Solid Edge part; units mm, degrees
sketch "Sketch1" plane through (0, 0, 0) normal (0, -1, 0) x (1, 0, 0)
  line L0 (-7, -6) -> (7, -6)
  line L1 (7, -6) -> (7, 6)
  line L2 (7, 6) -> (-7, 6)
  line L3 (-7, 6) -> (-7, -6)
  dimension "D1" = 7
  dimension "D2" = 7
extrude "Protrusion1" add sketch "Sketch1" along normal blind 40
sketch "Sketch2" plane through (0, -18, -6) normal (0, 0, -1) x (0, 1, 0)
  circle A0 centre (-15.5, 0) radius 6
  dimension "D1" = 15.5
extrude "Cutout1" cut sketch "Sketch2" against normal through all
sketch "Sketch3" plane through (7, -15, 0) normal (1, 0, 0) x (0, 1, 0)
  line L0 (-25, -2) -> (3, -2)
  line L1 (3, -2) -> (3, 6)
  dimension "D1" = 3
  dimension "D2" = 25
extrude "Cutout2" cut sketch "Sketch3" against normal through all material side at (7, -26, -1.95)
sketch "Sketch4" plane through (0, -18, -6) normal (0, 0, -1) x (0, 1, 0)
  line L0 (-10.3038, 3) -> (-8.3038, 3)
  arc A0 (-8.3038, 3) -> (-8.3038, -3) centre (-8.3038, 0) cw
  line L1 (-10.3038, -3) -> (-8.3038, -3)
  line L2 (-10.3038, 3) -> (-10.3038, -3)
  dimension "D1" = 10.3038
extrude "Cutout3" cut sketch "Sketch4" against normal through all
sketch "Sketch5" plane through (7, -20, 0) normal (1, 0, 0) x (0, -1, 0)
  line L0 (20, 2) -> (23, 2)
  line L1 (23, 2) -> (23, 27)
  line L2 (23, 27) -> (20, 27)
  line L3 (20, 27) -> (20, 2)
  dimension "D1" = 20
  dimension "D2" = 23
extrude "Protrusion2" add sketch "Sketch5" against normal up to vertex (14 mm away)
sketch "Sketch6" plane through (0, -23, -6) normal (0, 0, -1) x (0, -1, 0)
  line L0 (17, 6.5) -> (-7, 6.5)
  line L1 (-7, 6.5) -> (-7, -6.5)
  line L2 (-7, -6.5) -> (17, -6.5)
  line L3 (17, -6.5) -> (17, -7)
  line L4 (17, -7) -> (20, -7)
  line L5 (20, -7) -> (20, -9.5)
  line L6 (20, -9.5) -> (-10, -9.5)
  line L7 (-10, -9.5) -> (-10, 9.5)
  line L8 (-10, 9.5) -> (20, 9.5)
  line L9 (20, 9.5) -> (20, 7)
  line L10 (20, 7) -> (17, 7)
  line L11 (17, 7) -> (17, 6.5)
  dimension "D1" = 17
extrude "Protrusion3" add sketch "Sketch6" along normal up to vertex (21 mm away) and the other way up to vertex (4 mm away)
sketch "Sketch7" plane through (0, -43, -14.5) normal (0, -1, 0) x (-1, 0, 0)
  line L0 (-4, 4.5) -> (4, 4.5)
  line L1 (4, 4.5) -> (4, 12.5)
  line L2 (4, 12.5) -> (-4, 12.5)
  line L3 (-4, 12.5) -> (-4, 4.5)
  dimension "D1" = 4
  dimension "D2" = 4
extrude "Cutout4" cut sketch "Sketch7" against normal up to next
fillet "Verrundung_9" radius 3 2 edges at (4, -41.5, -19) (-4, -41.5, -19)
fillet "Verrundung_10" radius 3 5 edges at (0, -43, -19) (-3.1213, -43, -19.8787) (-4, -43, -24.5) (3.1213, -43, -19.8787) (4, -43, -24.5)
sketch "Sketch8" plane through (9.5, -28, -14.5) normal (1, 0, 0) x (0, 1, 0)
  line L0 (15, 12.5) -> (16, 12.5)
  line L1 (16, 12.5) -> (16, 20.5)
  line L2 (16, 20.5) -> (28, 20.5)
  line L3 (28, 20.5) -> (28, -4.5)
  line L4 (28, -4.5) -> (15, -4.5)
  line L5 (15, -4.5) -> (15, 12.5)
  dimension "D1" = 28
extrude "Protrusion4" add sketch "Sketch8" against normal up to vertex (19 mm away)
sketch "Sketch9" plane through (-9.5, -21.5, -10.5) normal (-1, 0, 0) x (0, 1, 0)
  arc A0 (13, -8.1957) -> (18, -8.1957) centre (15.5, -10.5) ccw
  line L0 (17.3, 4) -> (18, -8.1957)
  line L1 (13.7, 4) -> (17.3, 4)
  line L2 (13, -8.1957) -> (13.7, 4)
  dimension "D1" = 13.7
  dimension "D2" = 15.5
  dimension "D3" = 13
extrude "Extrusionsausschnitt_13" cut sketch "Sketch9" against normal blind 1.5
sketch "Sketch10" plane through (0, -6.5, -19) normal (0, 0, -1) x (0, 1, 0)
  line L0 (-6.5, 9.5) -> (-6.5, -1.5)
  line L1 (-6.5, -1.5) -> (6.5, -1.5)
extrude "Cutout5" cut sketch "Sketch10" against normal through all material side at (4, -12.95, -19)
sketch "Sketch11" plane through (-9.5, -21.5, -10.5) normal (-1, 0, 0) x (0, 0, 1)
  circle A0 centre (10.5, 15.5) radius 1.1
extrude "Cutout6" cut sketch "Sketch11" against normal through all
sketch "Sketch12" plane through (-1.5, -6.5, -6.5) normal (1, 0, 0) x (0, 1, 0)
  circle A0 centre (0.5, 6.5) radius 4
extrude "Extrusionsausschnitt_16" cut sketch "Sketch12" against normal blind 5
fillet "Verrundung_30" radius 2 3 edges at (9.5, -13, -14.5) (9.5, -43, -14.5) (-9.5, -43, -14.5)
fillet "Verrundung_31" radius 5 4 edges at (-5.5, -13, -19) (-5.5, 0, -19) (-5.5, 0, 6) (-5.5, -12, 6)
properties material "Nylon, allgemein"
Read the model definition and answer for the solid it produces. Units are mm, in the model's axes. A direction names the side the tool comes from. Round coordinates to 2 decimals unless told otherwise and drop trailing zeros. Write each loop counter-clockwise with the first axis right and the second up, starting at its lowest first coordinate (ties: lowest second). Pieces come first, ordered by that corner, then holes. Notation, with made-up numbers: M 68.25,57 L 81.25,57 A26 cw 81.25,82 Z; hole C 78,24.25 d4. An arc over 180 degrees is marked long. Use a Markdown table: item, result.
1) The part is cut by section B-B (z = 0). Write down the section's boundary in (x, y).
Answers follow:
| item | result |
|---|---|
| outline | M -9.5,-12 L -1.5,-12 L -1.5,-10 L -6.5,-10 L -6.5,-7.1 L -8,-7.1 L -8,-9.4 L -9.5,-9.4 Z; M -9.5,-2.6 L -8,-2.6 L -8,-4.9 L -6.5,-4.9 L -6.5,-2 L -1.5,-2 L -1.5,0 L -9.5,0 Z |
2) Straight lines are drawn through the part: line 1 along Y through (x, z) = (-7.05, 0); line 2 along Z through (x, y) = (-8.9, -6); line 3 along X through (y, z) = (-38, -13). For each, find the intervals that lie inside material, in ascending order. Write a range as [from, to].
Answers follow:
| item | result |
|---|---|
| line 1 | y = [-12, -7.1], [-4.9, 0] |
| line 2 | z = [-19, -14.5], [3.4, 6] |
| line 3 | x = [-9.5, -6.5], [6.5, 9.5] |
3) Flat-ended cylindrical pins translate along their axes: pin 1 (10.5 mm diameter, centred on x = 1, y = -34, fed in from -Z); pin 2 (3.5 mm diameter, centred on y = -6, z = 0, fed in from +X); pin 3 (0.9 mm diameter, centred on x = -6, z = 0, fed in from -Y). Find the tip coordinate at first contact, or state that the pin passes through.
Answers follow:
| item | result |
|---|---|
| pin 1 | stops at z = -6 |
| pin 2 | stops at x = -6.5 |
| pin 3 | stops at y = -12 |
4) The part is cut by section A-A (y = -27.5). Write down the section's boundary in (x, z).
Answers follow:
| item | result |
|---|---|
| outline | M -9.5,-27 L -6.5,-27 L -6.5,-6 L -3,-6 L -3,-2 L -9.5,-2 Z; M 3,-6 L 6.5,-6 L 6.5,-27 L 9.5,-27 L 9.5,-2 L 3,-2 Z |
5) A tool of negligible diameter and unlimited length cuts with its end or side. For faces 1 (the flat face through (-8.76, -3.855, -8.488)), 2 (the flat face through (-5, -6, -19)), 3 (the flat face through (-5, -12, -1)), 4 (the flat face through (6.5, -28, -16)), 5 (the cylindrical face through (-0.01, -42.1, -18.14)), from which of +Z, -Z, +X, -X, +Y, -Y can it reach the whole face along a straight path? Write none if from no direction.
Answers follow:
| item | result |
|---|---|
| face 1 | -X |
| face 2 | -Z, +X, -X, +Y |
| face 3 | +Z, +X, -X, -Y |
| face 4 | -Z |
| face 5 | -Z, -Y |
6) For a pull along Y with two mould halves and no side action, classify faces 6 (the flat face through (0, -40, -14)), 7 (the flat face through (9.5, -28, -14)), 8 (the flat face through (-3, -27, -4)), 9 (the flat face through (3, -13, -14)) as pulls with the +Y half, pulls with the -Y half, needs draft (parallel to the pull), parting line crosses it, or undercut.
Answers follow:
| item | result |
|---|---|
| face 6 | undercut |
| face 7 | needs draft |
| face 8 | undercut |
| face 9 | pulls with the +Y half |
